from build123d import *

# Parameters (mm, degrees)
BOSS_EXTRUDE1_DEPTH = 20
SKETCH3_W           = 36
SKETCH3_H           = 19
BOSS_EXTRUDE2_DEPTH = 3
FILLET3_R           = 9.5
FILLET4_R           = 9.5
SKETCH4_R           = 5
BOSS_EXTRUDE3_DEPTH = 4.24
SKETCH5_R           = 12
BOSS_EXTRUDE4_DEPTH = 2
SKETCH6_R           = 2.55
CUT_EXTRUDE4_DEPTH  = 46.01365694
SKETCH8_R           = 0.5
CUT_EXTRUDE5_DEPTH  = 2


with BuildPart() as part:
    # Sketch1 → Boss-Extrude1 (new body)
    with BuildSketch(Plane(origin=(0, 0, 0), x_dir=(1, 0, 0), z_dir=(0, 1, 0))):
        Polygon((20.135, 9.38), (26.635, 9.38), (26.635, 11.88), (20.135, 11.88), (20.135, 16.88), (-20.135, 16.88), (-20.135, 11.88), (-26.635, 11.88), (-26.635, 9.38), (-20.135, 9.38), (-20.135, -16.88), (20.135, -16.88), align=None)
    extrude(amount=BOSS_EXTRUDE1_DEPTH)

    # Sketch3 → Boss-Extrude2 (add)
    with BuildSketch(Plane(origin=(0, 0, -16.88), x_dir=(-1, 0, 0), z_dir=(0, 0, -1))):
        with Locations((0, 10)):
            Rectangle(SKETCH3_W, SKETCH3_H)
    extrude(amount=BOSS_EXTRUDE2_DEPTH)

    # Fillet3
    fillet3_edges = [part.edges().sort_by_distance(p)[0] for p in [
        (-18, 19.5, -18.38),
    ]]
    fillet(fillet3_edges, radius=FILLET3_R)

    # Fillet4
    fillet4_edges = [part.edges().sort_by_distance(p)[0] for p in [
        (-18, 0.5, -18.38),
    ]]
    fillet(fillet4_edges, radius=FILLET4_R - 0.0001)  # a hair under: the kernel refuses the full size

    # Sketch4 → Boss-Extrude3 (add)
    with BuildSketch(Plane(origin=(0, 0, -19.88), x_dir=(-1, 0, 0), z_dir=(0, 0, -1))):
        with Locations(Location((8.5, 10, 0), (0, 0, 180))):
            Circle(SKETCH4_R)
    extrude(amount=BOSS_EXTRUDE3_DEPTH)

    # Sketch5 → Boss-Extrude4 (add)
    with BuildSketch(Plane(origin=(0, 0, -24.12), x_dir=(-1, 0, 0), z_dir=(0, 0, -1))):
        with Locations((8.5, 10.128454218)):
            Circle(SKETCH5_R)
    extrude(amount=BOSS_EXTRUDE4_DEPTH)

    # Sketch6 → Cut-Extrude4 (cut, through all)
    with BuildSketch(Plane(origin=(0, 0, -11.88), x_dir=(-1, 0, 0), z_dir=(0, 0, -1))):
        with Locations((-24.135, 15.5)):
            Circle(SKETCH6_R)
        with Locations((-24.135, 4.5)):
            Circle(SKETCH6_R)
        with Locations((24.135, 15.5)):
            Circle(SKETCH6_R)
        with Locations((24.135, 4.5)):
            Circle(SKETCH6_R)
    extrude(amount=-CUT_EXTRUDE4_DEPTH, mode=Mode.SUBTRACT)

    # Sketch8 → Cut-Extrude5 (cut)
    with BuildSketch(Plane(origin=(0, 0, -26.12), x_dir=(-1, 0, 0), z_dir=(0, 0, -1))):
        with Locations((8.5, 10)):
            Circle(SKETCH8_R)
        with Locations((1.675504615, 11.557646538)):
            Circle(SKETCH8_R)
        with Locations((1.5, 10)):
            Circle(SKETCH8_R)
        with Locations((6.942353462, 16.824495385)):
            Circle(SKETCH8_R)
        with Locations((8.5, 17)):
            Circle(SKETCH8_R)
        with Locations((10.057646538, 16.824495385)):
            Circle(SKETCH8_R)
        with Locations((15.324495385, 11.557646538)):
            Circle(SKETCH8_R)
        with Locations((15.5, 10)):
            Circle(SKETCH8_R)
        with Locations((15.324495385, 8.442353462)):
            Circle(SKETCH8_R)
        with Locations((10.057646538, 3.175504615)):
            Circle(SKETCH8_R)
        with Locations((8.5, 3)):
            Circle(SKETCH8_R)
        with Locations((6.942353462, 3.175504615)):
            Circle(SKETCH8_R)
        with Locations((1.675504615, 8.442353462)):
            Circle(SKETCH8_R)
    extrude(amount=-CUT_EXTRUDE5_DEPTH, mode=Mode.SUBTRACT)


solid = part.part
Design review of the part built by this model. Coordinates are the model's own, in mm. A direction names the side the tool comes from. Give positions to 0.01 mm unless a question says otherwise; leave off trailing zeros. Order: outer loops, then holes, each group sorted by start corner. A loop starts at its lowest first (then second) coordinate and runs counter-clockwise, first axis right, second up. Notation, with made-up numbers: (31.25, 72) - (41.25, 72) arc R11 ccw to (41.25, 93) - close; hole circle Ø5 at (-39, -39.75). An arc over 180 degrees is marked (long way). Write item = value, one per line. Start each with the question number.
Q1. To check wall thickness, follow L1, parallel to Z at x = -17, y = 14.75; L2, parallel to Z at x = -12, y = 2.5; L3, parallel to Y at x = -15, z = 7. State the ranges of each line that lie inside material, in increasing order. Write a range as from..to.
Q2. Mouldability with a two-part tool opening along Z and no side actions: class faces 1 (the face through (-14, 10, -24.12)), 2 (the face through (-21.587, 15.605, -10.648)), 3 (the face through (23, 10, -9.38)) as released by +Z, released by -Z, zero draft, split by the parting line, or undercut.
Q3. We need section A-A on x = 22.5. State the section outline as (y, z) points, plus the area to 3 significant figures.
Q4. Clearance check with flat-ended pins moving along their axes: pin 1 Ø0.9 at (y, z) = (9.5, -18.5) entering from +X; pin 2 Ø6 at (y, z) = (12.5, 7) entering from -X (3 decimals); pin 3 Ø5 at (x, y) = (22, 5.5) entering from -Z; pin 4 Ø3 at (x, y) = (-24.135, 15.5) entering from +Z. State where each tip first meets the part, or that it passes through.
Q5. We need section D-D on x = -11.5. State the section outline as (y, z) points.
Q6. We need section C-C on x = 2.5. State the section outline as (y, z) points.
Q7. Tool access review of faces 4 (the face through (-3.73, 8.5, -21.97)), 5 (the face through (-15.291, 3.357, -18.401)), 6 (the face through (-15.143, 16.791, -18.401)), 7 (the face through (20.135, 10, -14)), 8 (the face through (20.135, 10, 4)): name each direction out of +Z, -Z, +X, -X, +Y, -Y from which nothing blocks a thin tool from reaching the whole face with its end or side.
Working result:
q1.L1 = -26.12..-24.12, -16.88..16.88
q1.L2 = -26.12..-24.12, -19.88..16.88
q1.L3 = 0..20
q2.face_1 = undercut
q2.face_2 = zero draft
q2.face_3 = released by +Z
q3.outline = (0, -11.88) - (2.54, -11.88) - (2.54, -9.38) - (0, -9.38) - close; (6.46, -11.88) - (13.54, -11.88) - (13.54, -9.38) - (6.46, -9.38) - close; (17.46, -11.88) - (20, -11.88) - (20, -9.38) - (17.46, -9.38) - close
q3.area = 30.4 mm²
q4.pin_1 = 18
q4.pin_2 = -20.135
q4.pin_3 = -16.88
q4.pin_4 = through
q5.outline = (-1.49, -26.12) - (21.75, -26.12) - (21.75, -24.12) - (14, -24.12) - (14, -19.88) - (19.01, -19.88) - (19.01, -16.88) - (20, -16.88) - (20, 16.88) - (0, 16.88) - (0, -16.88) - (0.99, -16.88) - (0.99, -19.88) - (6, -19.88) - (6, -24.12) - (-1.49, -24.12) - close
q6.outline = (0, -16.88) - (0.5, -16.88) - (0.5, -19.88) - (19.5, -19.88) - (19.5, -16.88) - (20, -16.88) - (20, 16.88) - (0, 16.88) - close; (5.33, -26.12) - (14.92, -26.12) - (14.92, -24.12) - (5.33, -24.12) - close
q7.face_4 = none
q7.face_5 = -X, -Y
q7.face_6 = -X, +Y
q7.face_7 = -Z, +X, +Y, -Y
q7.face_8 = +Z, +X, +Y, -Y
